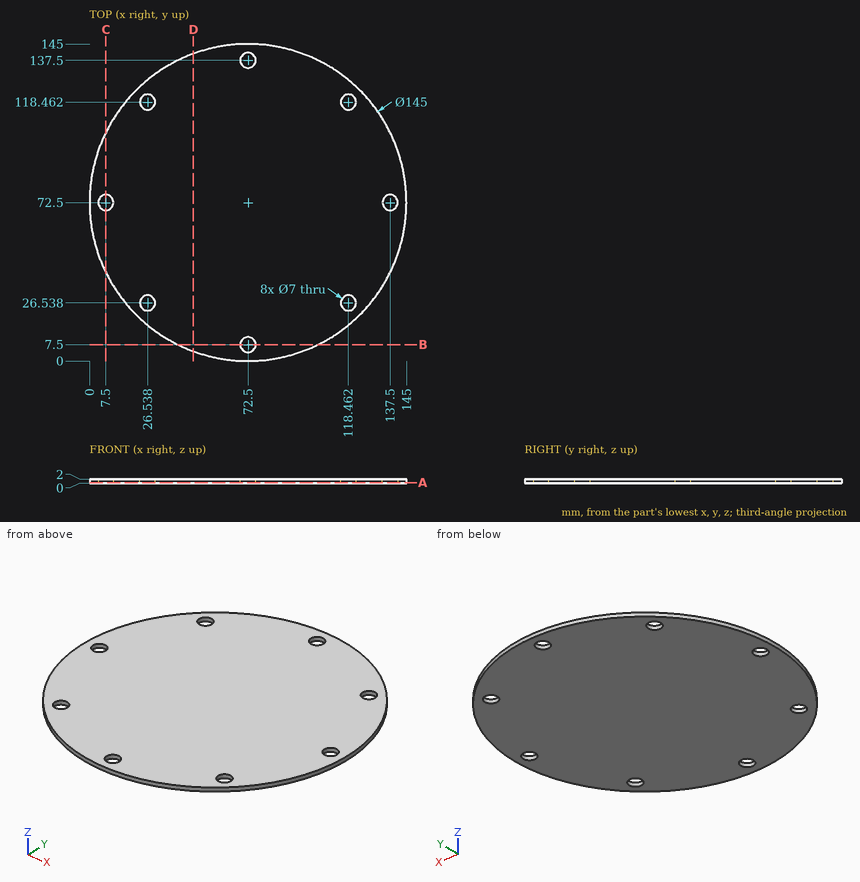
For this review, use the dimensioned drawing (mm, ordinates from the lowest corner) and the shaded views. Coordinates: 2 decimals unless noted, no trailing zeros. Order: outer loops, then holes, each group sorted by start corner. A loop starts at its lowest first (then second) coordinate and runs counter-clockwise, first axis right, second up. Notation, with made-up numbers: (63, 73) - (71, 73) arc R20 cw to (71, 87) - close; hole circle Ø1 at (-19.75, 5.5). An arc over 180 degrees is marked (long way). Answer in a Markdown table with one row per item.
(1) Clearance check with flat-ended pins moving along their axes: pin 1 (6.5 mm diameter, centred on x = 7.5, y = 72.5, fed in from -Z); pin 2 (1 mm diameter, centred on y = 126.5, z = 1.5, fed in from +X). State where each tip first meets the part, or that it passes through.
Checked values:
| item | result |
|---|---|
| pin 1 | through |
| pin 2 | x = 121.43 |
(2) Wall thickness on line 1 along Y through (x, z) = (117, 1.35); line 2 along Y through (x, z) = (7.5, 1.5); line 3 along Y through (x, z) = (138, 1.5): over which ranges is each line inside the solid? List them lowest first. Write a range as from..to.
Checked values:
| item | result |
|---|---|
| line 1 | 15.26..23.36, 29.72..115.28, 121.64..129.74 |
| line 2 | 40.39..69, 76..104.61 |
| line 3 | 41.42..69.04, 75.96..103.58 |
(3) Consider section D-D on x = 47.5. State the section outline as (y, z) points.
Checked values:
| item | result |
|---|---|
| outline | (4.45, 0) - (140.55, 0) - (140.55, 2) - (4.45, 2) - close |
(4) Consider section A-A on z = 0.35. Give the number of separate pieces and of enclosed holes in the cut face, plus the area to 3 significant figures.
Checked values:
| item | result |
|---|---|
| separate pieces | 1 |
| enclosed holes | 8 |
| area | 16,200 mm^2 |
(5) Consider section B-B on y = 7.5. State the section outline as (x, z) points, plus the area to 3 significant figures.
Checked values:
| item | result |
|---|---|
| outline | (40.39, 0) - (69, 0) - (69, 2) - (40.39, 2) - close; (76, 0) - (104.61, 0) - (104.61, 2) - (76, 2) - close |
| area | 114 mm^2 |
